```python
from build123d import *

# Parameters (mm, degrees)
BOSS_EXTRUDE1_DEPTH      = 190
SKETCH2_R                = 2.1
CUT_EXTRUDE1_DEPTH       = 193.574660846
CUT_EXTRUDE3_START       = -29
CUT_EXTRUDE3_DEPTH       = 29
FILLET1_R                = 2
CUT_EXTRUDE4_DEPTH       = 22
CUT_EXTRUDE5_REACH       = 183.805
SKETCH5_R                = 2.05
CUT_EXTRUDE6_START       = -4
CUT_EXTRUDE6_DEPTH       = 7.5
SKETCH6_R                = 2
BOSS_EXTRUDE2_DEPTH      = 2
CHAMFER1_SIZE            = 0.5
CHAMFER1_OF_MIRROR1_SIZE = 0.5
FILLET2_R                = 2


# Read off the part's stored shape, not the designer's step: Cut-Extrude3
with BuildPart() as part:
    # Sketch1 → Boss-Extrude1 (new body)
    with BuildSketch(Plane(origin=(0, 0, 0), x_dir=(0, 0, -1), z_dir=(1, 0, 0))):
        Polygon((-3, 6), (-3, 35), (12, 35), (12, 21.281778339), (12, 18), (12, 6), align=None)
    extrude(amount=BOSS_EXTRUDE1_DEPTH)

    # Sketch2 → Cut-Extrude1 (cut, through all)
    with BuildSketch(Plane(origin=(0, 35, 0), x_dir=(1, 0, 0), z_dir=(0, 1, 0))):
        with Locations(Location((160, 5, 0), (0, 0, 270))):
            Circle(SKETCH2_R)
        with Locations(Location((30, 5, 0), (0, 0, 270))):
            Circle(SKETCH2_R)
    extrude(amount=-CUT_EXTRUDE1_DEPTH, mode=Mode.SUBTRACT)

    # Cut-Extrude3 outline → Cut-Extrude3 (cut)
    with BuildSketch(Plane(origin=(0, 35, 0), x_dir=(1, 0, 0), z_dir=(0, 1, 0)).offset(CUT_EXTRUDE3_START)):
        with BuildLine():
            ThreePointArc((23, 5), (25.050252532, 9.949747468), (30, 12))
            Line((30, 12), (10, 12))
            Line((10, 12), (10, 5))
            Line((10, 5), (23, 5))
        make_face()
        with BuildLine():
            Line((180, 12), (160, 12))
            ThreePointArc((160, 12), (164.949747468, 9.949747468), (167, 5))
            Line((167, 5), (180, 5))
            Line((180, 5), (180, 12))
        make_face()
        with BuildLine():
            Line((37, 5), (153, 5))
            ThreePointArc((153, 5), (155.050252532, 9.949747468), (160, 12))
            Line((160, 12), (30, 12))
            ThreePointArc((30, 12), (34.949747468, 9.949747468), (37, 5))
        make_face()
    extrude(amount=CUT_EXTRUDE3_DEPTH, mode=Mode.SUBTRACT)

    # Fillet1
    fillet1_edges = [part.edges().sort_by_distance(p)[0] for p in [
        (10, 20.5, -5),
        (180, 20.5, -5),
    ]]
    fillet(fillet1_edges, radius=FILLET1_R)

    # Sketch4 → Cut-Extrude4 (cut)
    with BuildSketch(Plane.XZ.offset(-6)):
        Polygon((34.151410886, -4.276672839), (31.885792779, -0.8604896), (27.794482256, -1.114480816), (25.968789841, -4.784655272), (28.234407948, -8.200838512), (32.325718471, -7.946847295), align=None)
        Polygon((164.091310523, -4.746008784), (161.825692416, -1.329825544), (157.734381893, -1.583816761), (155.908689477, -5.253991216), (158.174307584, -8.670174456), (162.265618107, -8.416183239), align=None)
    extrude(amount=-CUT_EXTRUDE4_DEPTH, mode=Mode.SUBTRACT)

    # Sketch5 → Cut-Extrude5 (cut, up to next)
    with BuildSketch(Plane(origin=(178, 0, 0), x_dir=(0, 0, -1), z_dir=(1, 0, 0)), mode=Mode.PRIVATE) as cut_extrude5_sk1:
        with Locations(Location((5, 23, 0), (0, 0, 270))):
            Circle(SKETCH5_R)
    cut_extrude5_tool1 = extrude(cut_extrude5_sk1.sketch, amount=CUT_EXTRUDE5_REACH, mode=Mode.PRIVATE) & part.part
    cut_extrude5 = cut_extrude5_tool1.solids().sort_by_distance((178, 23, -5))[0]
    add(cut_extrude5, mode=Mode.SUBTRACT)

    # Sketch5<3> → Cut-Extrude6 (cut)
    with BuildSketch(Plane(origin=(178, 0, 0), x_dir=(0, 0, -1), z_dir=(1, 0, 0)).offset(CUT_EXTRUDE6_START)):
        Polygon((5, 18.900813089), (8.55, 20.950406544), (8.55, 25.049593456), (5, 27.099186911), (1.45, 25.049593456), (1.45, 20.950406544), align=None)
    cut_extrude6 = extrude(amount=CUT_EXTRUDE6_DEPTH, mode=Mode.SUBTRACT)

    # Sketch6 → Boss-Extrude2 (add)
    with BuildSketch(Plane(origin=(190, 0, 0), x_dir=(0, 0, -1), z_dir=(1, 0, 0))):
        with Locations((5, 13)):
            Circle(SKETCH6_R)
    boss_extrude2 = extrude(amount=BOSS_EXTRUDE2_DEPTH)

    # Chamfer1
    chamfer1_edges = [part.edges().sort_by_distance(p)[0] for p in [
        (192, 13, -3),
    ]]
    chamfer(chamfer1_edges, length=CHAMFER1_SIZE)

    # Mirror1: Cut-Extrude5, Cut-Extrude6, Boss-Extrude2 across plane
    add(cut_extrude5.mirror(Plane(origin=(95, 0, 0), x_dir=(0, 0, 1), z_dir=(1, 0, 0))), mode=Mode.SUBTRACT)
    add(cut_extrude6.mirror(Plane(origin=(95, 0, 0), x_dir=(0, 0, 1), z_dir=(1, 0, 0))), mode=Mode.SUBTRACT)
    add(boss_extrude2.mirror(Plane(origin=(95, 0, 0), x_dir=(0, 0, 1), z_dir=(1, 0, 0))))

    # Chamfer1 of Mirror1
    chamfer1_of_mirror1_edges = [part.edges().sort_by_distance(p)[0] for p in [
        (-2, 13, -3),
    ]]
    chamfer(chamfer1_of_mirror1_edges, length=CHAMFER1_OF_MIRROR1_SIZE)

    # Fillet2
    fillet2_edges = [part.edges().sort_by_distance(p)[0] for p in [
        (185, 6, -12),
        (95, 6, 3),
        (153, 20.5, -5),
        (37, 20.5, -5),
        (164.949747468, 6, -9.949747468),
        (95, 6, -5),
        (34.949747468, 6, -9.949747468),
        (5, 6, -12),
        (23, 20.5, -5),
        (10, 6, -9.5),
        (10, 20.5, -12),
        (167, 20.5, -5),
        (180, 20.5, -12),
        (180, 6, -9.5),
        (17.5, 6, -5),
        (172.5, 6, -5),
        (10.585786438, 6, -5.585786438),
        (179.414213562, 6, -5.585786438),
    ]]
    fillet(fillet2_edges, radius=FILLET2_R)


solid = part.part
```
Geometry check sheet. Reference: the model listing, model coordinates, mm. A direction names the side the tool comes from. Coordinates: 2 decimals unless noted, no trailing zeros. Write each loop counter-clockwise with the first axis right and the second up, starting at its lowest first coordinate (ties: lowest second). Pieces come first, ordered by that corner, then holes. Notation, with made-up numbers: M 0.5,-22 L 52.5,-22 A27 ccw 52.5,7 Z; hole C 33.5,79 d4. An arc over 180 degrees is marked long. Answer as a JSON object with one key per item and string values.
1. Go/stop test with flat-tipped pins: pin 1 Ø6 at (x, y) = (152, 15.5) entering from -Z; pin 2 Ø4 at (y, z) = (11, -8.5) entering from -X; pin 3 Ø2 at (x, z) = (161.5, -5.5) entering from -Y; pin 4 Ø2.5 at (x, z) = (160, -5) entering from -Y. Record where each tip stops, or that it passes through.
Answers below:
{"pin 1": "stops at z = -9.9", "pin 2": "stops at x = 0", "pin 3": "stops at y = 28", "pin 4": "passes through"}
2. Tool access check on faces 4 (the flat face through (157, 16.8, -6.9)), 5 (the flat face through (174, 23, -4)), 6 (the flat face through (180, 21, -9)), 7 (the flat face through (180.5, 19.91, -6.75)), 8 (the cylindrical face through (185.69, 24.627, -3.753)). Record the directions out of +Z, -Z, +X, -X, +Y, -Y that give a thin tool (end or side, any length) a straight path to the whole face; none if there is none.
Answers below:
{"face 4": "-Y", "face 5": "-Z", "face 6": "-Z, +Y, -Y", "face 7": "none", "face 8": "+X"}
3. Section check B-B, the plane x = 89. Enter the section's corners in (y, z).
Answers below:
{"outline": "M 6,-3 A2 ccw 8,-5 L 35,-5 L 35,3 L 8,3 A2 ccw 6,1 Z"}
4. Draft check along Y on faces 1 (the cylindrical face through (190.74, 14.352, -3.526)), 2 (the flat face through (177.7, 26.09, -3.25)), 3 (the flat face through (27.086, 16.846, -6.469)). Enter one of: released by +Y, released by -Y, zero draft, split by the parting line, or undercut.
Answers below:
{"face 1": "split by the parting line", "face 2": "undercut", "face 3": "zero draft"}
5. Scan lines: L1, parallel to Z at x = 160, y = 32.75; L2, parallel to X at y = 33.5, z = -9.25; L3, parallel to X at y = 15.5, z = -4. Record each from-to range of solid material in increasing order.
Answers below:
{"L1": "z = -12 to -7.1, -2.9 to 3", "L2": "x = 0 to 10, 24.44 to 35.56, 154.44 to 165.56, 180 to 190", "L3": "x = 0 to 26.36, 33.97 to 156.53, 163.6 to 190"}
6. Section check A-A, the plane y = 23. Give the number of separate pieces and of enclosed holes in the cut face, plus the area to 3 significant figures.
Answers below:
{"separate pieces": "3", "enclosed holes": "2", "area": "1,590 mm²"}
